from build123d import *

# Parameters (mm, degrees)
F0_W           = 381
F0_H           = 381
F1_DEPTH       = 381
F3_D           = 6.35
F3_CSINK_D     = 12.7
F3_CSINK_ANGLE = 90
F4_R           = 66.123945
F5_DEPTH       = 50


with BuildPart() as f1:
    # F0 (on Front) → F1 (new body)
    with BuildSketch(Plane.XZ):
        with Locations((190.5, 190.5)):
            Rectangle(F0_W, F0_H)
    extrude(amount=F1_DEPTH)

    # F3 (through all)
    with Locations(Plane.XZ.offset(381)):
        with Locations((123.825006, 267.081022)):
            CounterSinkHole(F3_D / 2, F3_CSINK_D / 2, counter_sink_angle=F3_CSINK_ANGLE)

    # F4 (on face) → F5 (join)
    with BuildSketch(Plane.YZ.offset(381)):
        with Locations((-141.749784, 196.200415)):
            Circle(F4_R)
    extrude(amount=F5_DEPTH)


solid = f1.part
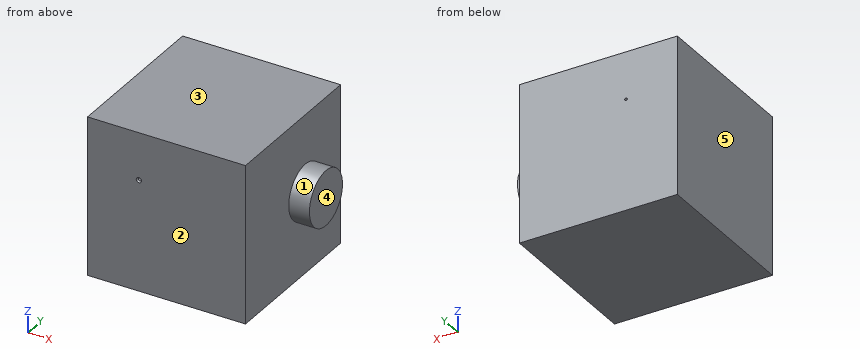
Part model, mm, in its own coordinate system. Face numbers are marked on the shaded views. A direction names the side the tool comes from. Give positions to 0.01 mm unless a question says otherwise; leave off trailing zeros. Loops run counter-clockwise (first coordinate to the right, second up) from the corner with the lowest first, then second, coordinate; pieces in that order, holes last. Notation, with made-up numbers: M 17,-24.75 L 67,-24.75 A27 ccw 67,5.25 Z; hole C 83.5,89.5 d7. An arc over 180 degrees is marked long. Put each result on its own line as item: value. Start each with the question number.
1) Flat gauge pin, fed straight in: pin 1 (6 mm diameter, centred on y = -269, z = 256, fed in from +X). Where does the tip first touch, or does it go through?
2) 3-axis set-ups, long thin cutter, end or side, ignore diameter. For the marked faces 1 and 2: which of +Z, -Z, +X, -X, +Y, -Y reach the whole face in a straight line?
3) Pull direction X, two halves, no side cores. Call the marked faces 3, 4 and 5: +X half, -X half, draft (parallel to the pull), parting line (faces both ways), or undercut.
4) Saw through at C-C (y = -167). List the corners of the cut face in (x, z) (3 decimals), then the cut area to 3 significant figures.
5) Saw through at A-A (y = -107.5). List the corners of the cut face in (x, z) (3 decimals).
6) Probe probe 1 along X at (y, z) = (-266.5, 272.5). List the from-to ranges inside material, lowest first.
7) Saw through at D-D (x = 396.5). List the corners of the cut face in (y, z), then the cut area to 3 significant figures.
8) Saw through at B-B (z = 253.5). List the corners of the cut face in (x, y).
Numbers:
1. pin 1: x = 381
2. face 1: +X
2. face 2: +Z, -Z, +X, -X, -Y
3. face 3: draft
3. face 4: +X half
3. face 5: -X half
4. outline: M 0,0 L 381,0 L 381,135.087 L 431,135.087 L 431,257.313 L 381,257.313 L 381,381 L 0,381 Z; hole C 123.825,267.081 d6.35
4. area: 151,000 mm^2
5. outline: M 0,0 L 381,0 L 381,139.638 L 431,139.638 L 431,252.763 L 381,252.763 L 381,381 L 0,381 Z; hole C 123.825,267.081 d6.35
6. probe 1: 0 to 381
7. outline: C -141.75,196.2 d132.25
7. area: 13,700 mm^2
8. outline: M 0,-381 L 381,-381 L 381,-174.75 L 431,-174.75 L 431,-108.75 L 381,-108.75 L 381,0 L 0,0 Z
